Geometry: final body of the model. Coordinates: model frame, mm. A direction names the side the tool comes from. Give positions to 0.01 mm unless a question says otherwise; leave off trailing zeros. Order: outer loops, then holes, each group sorted by start corner. A loop starts at its lowest first (then second) coordinate and runs counter-clockwise, first axis right, second up. Notation, with made-up numbers: (44.25, 64) - (59.25, 64) arc R29 cw to (59.25, 96) - close; hole circle Ø9 at (38.5, 40.25). An arc over 180 degrees is marked (long way). Put each result on its own line as item: value. Start each with the question number.
1. Set-up query: faces 5 (the flat face through (-28, 0, 12)), 6 (the flat face through (-1, 20, 57)). Return all of +Z, -Z, +X, -X, +Y, -Y with unobstructed straight access to the full face (end or side cutting, diameter ignored); none if empty.
2. Section D-D on x = -36. Return the cut outline in (y, z).
3. Ray query, line 1 along Y through (x, z) = (53, 59.3); line 2 along Y through (x, z) = (31, 48.5); line 3 along Z through (x, y) = (47, 6.5). Return the intervals inside material, ascending. Write a range as from..to.
4. Section C-C on x = 10.5. Return the cut outline in (y, z).
5. Section A-A on z = 15. Return the cut outline in (x, y), plus the area to 3 significant figures.
6. Section B-B on x = -53. Return the cut outline in (y, z), plus the area to 3 significant figures.
7. First-contact query: P1, Ø4, axis at x = 42.5, y = 21, coming from the -Z side; P2, Ø3.5, axis at x = -28.95, z = 33.05, coming from the +Y side. Flat tips, straight axial feed; report the tip coordinate or a pass-through.
8. Mould query, pull axis Z, two halves, no side actions, for faces 1 (the cylindrical face through (-2.354, 1.479, -43.225)), 2 (the cylindrical face through (-27.78, 1.48, 32.2)), 3 (the flat face through (-1, 19, 60)), 4 (the cylindrical face through (-53, 29, 58)). Classes: pulls with the +Z half, pulls with the -Z half, needs draft (parallel to the pull), parting line crosses it, or undercut.
from build123d import *

# Parameters (mm, degrees)
BOSS_EXTRUDE1_DEPTH = 3
SKETCH2_W           = 3
SKETCH2_H           = 35
BOSS_EXTRUDE2_DEPTH = 120
SKETCH3_R           = 2
CUT_EXTRUDE1_DEPTH  = 10


with BuildPart() as part:
    # Sketch1 → Boss-Extrude1 (new body)
    with BuildSketch(Plane(origin=(0, 0, 0), x_dir=(1, 0, 0), z_dir=(0, 1, 0))):
        with BuildLine():
            ThreePointArc((60, 0), (0, 60), (-60, 0))
            Line((-60, 0), (-60, -60))
            Line((-60, -60), (60, -60))
            Line((60, -60), (60, 0))
        make_face()
        with BuildLine():
            ThreePointArc((-28.86964292, -34.498602179), (-30.402233374, -33.136190163), (-29.039821358, -31.603599709))
            ThreePointArc((-29.039821358, -31.603599709), (-27.507230904, -32.966011725), (-28.86964292, -34.498602179))
        make_face(mode=Mode.SUBTRACT)
        with BuildLine():
            ThreePointArc((-43.727439791, -3.851425062), (-45.260030245, -2.489013046), (-43.89761823, -0.956422592))
            ThreePointArc((-43.89761823, -0.956422592), (-42.365027776, -2.318834608), (-43.727439791, -3.851425062))
        make_face(mode=Mode.SUBTRACT)
        with BuildLine():
            ThreePointArc((3.137054327, -42.768377551), (4.669644781, -44.130789567), (3.307232765, -45.663380021))
            ThreePointArc((3.307232765, -45.663380021), (1.774642311, -44.300968005), (3.137054327, -42.768377551))
        make_face(mode=Mode.SUBTRACT)
        with BuildLine():
            ThreePointArc((32.289465784, -26.581793404), (33.822056238, -27.944205419), (32.459644223, -29.476795874))
            ThreePointArc((32.459644223, -29.476795874), (30.927053769, -28.114383858), (32.289465784, -26.581793404))
        make_face(mode=Mode.SUBTRACT)
        with BuildLine():
            ThreePointArc((-31.06789629, 26.996663347), (-32.600486744, 28.359075363), (-31.238074729, 29.891665817))
            ThreePointArc((-31.238074729, 29.891665817), (-29.705484275, 28.529253801), (-31.06789629, 26.996663347))
        make_face(mode=Mode.SUBTRACT)
        with BuildLine():
            ThreePointArc((-2.085663271, 46.078249964), (-0.553072817, 44.715837949), (-1.915484832, 43.183247495))
            ThreePointArc((-1.915484832, 43.183247495), (-3.448075286, 44.54565951), (-2.085663271, 46.078249964))
        make_face(mode=Mode.SUBTRACT)
        with BuildLine():
            ThreePointArc((29.082980246, 9.659105906), (10.062455681, -28.264760528), (-27.861410752, -9.244235963))
            ThreePointArc((-27.861410752, -9.244235963), (-8.840886187, 28.679630471), (29.082980246, 9.659105906))
        make_face(mode=Mode.SUBTRACT)
        with BuildLine():
            ThreePointArc((44.949009286, 4.266295005), (46.48159974, 2.90388299), (45.119187724, 1.371292536))
            ThreePointArc((45.119187724, 1.371292536), (43.58659727, 2.733704551), (44.949009286, 4.266295005))
        make_face(mode=Mode.SUBTRACT)
        with BuildLine():
            ThreePointArc((30.261390853, 32.018469652), (28.728800399, 33.380881668), (30.091212414, 34.913472122))
            ThreePointArc((30.091212414, 34.913472122), (31.623802868, 33.551060107), (30.261390853, 32.018469652))
        make_face(mode=Mode.SUBTRACT)
    extrude(amount=BOSS_EXTRUDE1_DEPTH)

    # Sketch2 → Boss-Extrude2 (add)
    with BuildSketch(Plane.ZY.offset(60)):
        with Locations((58.5, 20.5)):
            Rectangle(SKETCH2_W, SKETCH2_H)
    extrude(amount=-BOSS_EXTRUDE2_DEPTH)

    # Sketch3 → Cut-Extrude1 (cut)
    with BuildSketch(Plane(origin=(0, 0, 57), x_dir=(-1, 0, 0), z_dir=(0, 0, -1))):
        with Locations((-53, 31)):
            Circle(SKETCH3_R)
        with Locations((53, 31)):
            Circle(SKETCH3_R)
        with Locations((53, 10)):
            Circle(SKETCH3_R)
        with Locations((-53, 10)):
            Circle(SKETCH3_R)
    extrude(amount=-CUT_EXTRUDE1_DEPTH, mode=Mode.SUBTRACT)


solid = part.part
Resolved:
1. face 5: +Z, -Z, +X, -X, -Y
1. face 6: -Z, +X, -X, +Y
2. outline: (0, -48) - (3, -48) - (3, 57) - (38, 57) - (38, 60) - (0, 60) - close
3. line 1: 0..8, 12..29, 33..38
3. line 2: 0..3
3. line 3: 57..60
4. outline: (0, -59.07) - (3, -59.07) - (3, -28.53) - (0, -28.53) - close; (0, 28.12) - (3, 28.12) - (3, 57) - (38, 57) - (38, 60) - (0, 60) - close
5. outline: (-60, 0) - (-25.25, 0) - (-25.25, 3) - (-60, 3) - close; (26.47, 0) - (60, 0) - (60, 3) - (26.47, 3) - close
5. area: 205 mm^2
6. outline: (0, -28.12) - (3, -28.12) - (3, 57) - (8, 57) - (8, 60) - (0, 60) - close; (12, 57) - (29, 57) - (29, 60) - (12, 60) - close; (33, 57) - (38, 57) - (38, 60) - (33, 60) - close
6. area: 345 mm^2
7. P1: z = 57
7. P2: y = 3
8. face 1: undercut
8. face 2: undercut
8. face 3: pulls with the +Z half
8. face 4: needs draft
